Read the model definition and answer for the solid it produces. Units are mm, in the model's axes. A direction names the side the tool comes from. Round coordinates to 2 decimals unless told otherwise and drop trailing zeros. Write each loop counter-clockwise with the first axis right and the second up, starting at its lowest first coordinate (ties: lowest second). Pieces come first, ordered by that corner, then holes. Notation, with made-up numbers: (-26.5, 77.5) - (27.5, 77.5) arc R18 ccw to (27.5, 98.5) - close; hole circle Ø10 at (-40, 72.5). An arc over 180 degrees is marked (long way). Answer as CSV lines item,"result". Start each with the question number.
1) Consider line 1 along X through (y, z) = (78, -47) (3 decimals); line 2 along Z through (x, y) = (9, 22) (3 decimals); line 3 along Z through (x, y) = (11, 110.5) (3 decimals). Determine where each line is inside the solid, lowest interval first.
2) For a pull along Z with two mould halves and no side action, classify faces 3 (the flat face through (13, 63, 0)), 4 (the flat face through (25.4, 48, -25)), 5 (the flat face through (13, 39, -47.625)), 6 (the flat face through (23, 102, -25)) as +Z half, -Z half, draft (parallel to the pull), parting line (faces both ways), or undercut.
3) Find section D-D on y = 94. Determine the outline of the cut face in (x, z) (3 decimals).
4) Find section B-B on x = 6.25. Determine the outline of the cut face in (y, z) (3 decimals), then the cut area to 3 significant figures.
5) Which of the six approach directions +Z, -Z, +X, -X, +Y, -Y give full straight-line access (tool end or side, diameter ignored) to faces 1 (the flat face through (13, 61, -3.175)), 2 (the flat face through (13, 38, -50.8))?
6) Find section A-A on z = -30. Determine the outline of the cut face in (x, y) (3 decimals).
7) Find section C-C on y = 14. Determine the outline of the cut face in (x, z) (3 decimals).
8) This flat-tipped pin is pushed along its axis until it touches: pin 1 (4 mm diameter, centred on x = 6, y = 113.5, fed in from -Z) (3 decimals). Where does it stop, or does it pass through?
from build123d import *

# Parameters (mm, degrees)
SKETCH1_W           = 25.4
SKETCH1_H           = 50.8
SKETCH1_W_2         = 19.05
SKETCH1_H_2         = 44.45
BOSS_EXTRUDE1_DEPTH = 127
CUT_EXTRUDE1_DEPTH  = 127


with BuildPart() as part:
    # Sketch1 → Boss-Extrude1 (new body)
    with BuildSketch(Plane(origin=(0, 0, 0), x_dir=(1, 0, 0), z_dir=(0, 1, 0))):
        with Locations((12.7, 25.4)):
            Rectangle(SKETCH1_W, SKETCH1_H)
        with Locations((12.7, 25.4)):
            Rectangle(SKETCH1_W_2, SKETCH1_H_2, mode=Mode.SUBTRACT)
    extrude(amount=BOSS_EXTRUDE1_DEPTH)

    # Sketch2 → Cut-Extrude1 (cut)
    with BuildSketch(Plane(origin=(25.4, 0, 0), x_dir=(0, 0, -1), z_dir=(1, 0, 0))):
        Polygon((0, 127), (50.8, 76.2), (50.8, 127), align=None)
    extrude(amount=-CUT_EXTRUDE1_DEPTH, mode=Mode.SUBTRACT)


solid = part.part
Check values:
1,line 1,"x = 0 to 3.175, 22.225 to 25.4"
1,line 2,"z = -50.8 to -47.625, -3.175 to 0"
1,line 3,"z = -3.175 to 0"
2,face 3,"+Z half"
2,face 4,"draft"
2,face 5,"undercut"
2,face 6,"-Z half"
3,outline,"(0, -33) - (3.175, -33) - (3.175, -3.175) - (22.225, -3.175) - (22.225, -33) - (25.4, -33) - (25.4, 0) - (0, 0) - close"
4,outline,"(0, -50.8) - (76.2, -50.8) - (79.375, -47.625) - (0, -47.625) - close; (0, -3.175) - (123.825, -3.175) - (127, 0) - (0, 0) - close"
4,area,"645 mm^2"
5,face 1,"+Y, -Y"
5,face 2,"-Z, +X, -X, +Y, -Y"
6,outline,"(0, 0) - (3.175, 0) - (3.175, 97) - (0, 97) - close; (22.225, 0) - (25.4, 0) - (25.4, 97) - (22.225, 97) - close"
7,outline,"(0, -50.8) - (25.4, -50.8) - (25.4, 0) - (0, 0) - close; hole (3.175, -47.625) - (22.225, -47.625) - (22.225, -3.175) - (3.175, -3.175) - close"
8,pin 1,"stops at z = -3.175"
